Here's the drawing with two shaded views (mm, measured from the low corner). I have some questions. A direction names the side the tool comes from. Coordinates: 2 decimals unless noted, no trailing zeros. Write each loop counter-clockwise with the first axis right and the second up, starting at its lowest first coordinate (ties: lowest second). Pieces come first, ordered by that corner, then holes. Notation, with made-up numbers: (0.25, 20.5) -> (43.25, 20.5) arc R3 ccw to (43.25, 24.5) -> close; hole circle Ø4 at (33.5, 72). An arc over 180 degrees is marked (long way). Put each result on its own line as item: value.
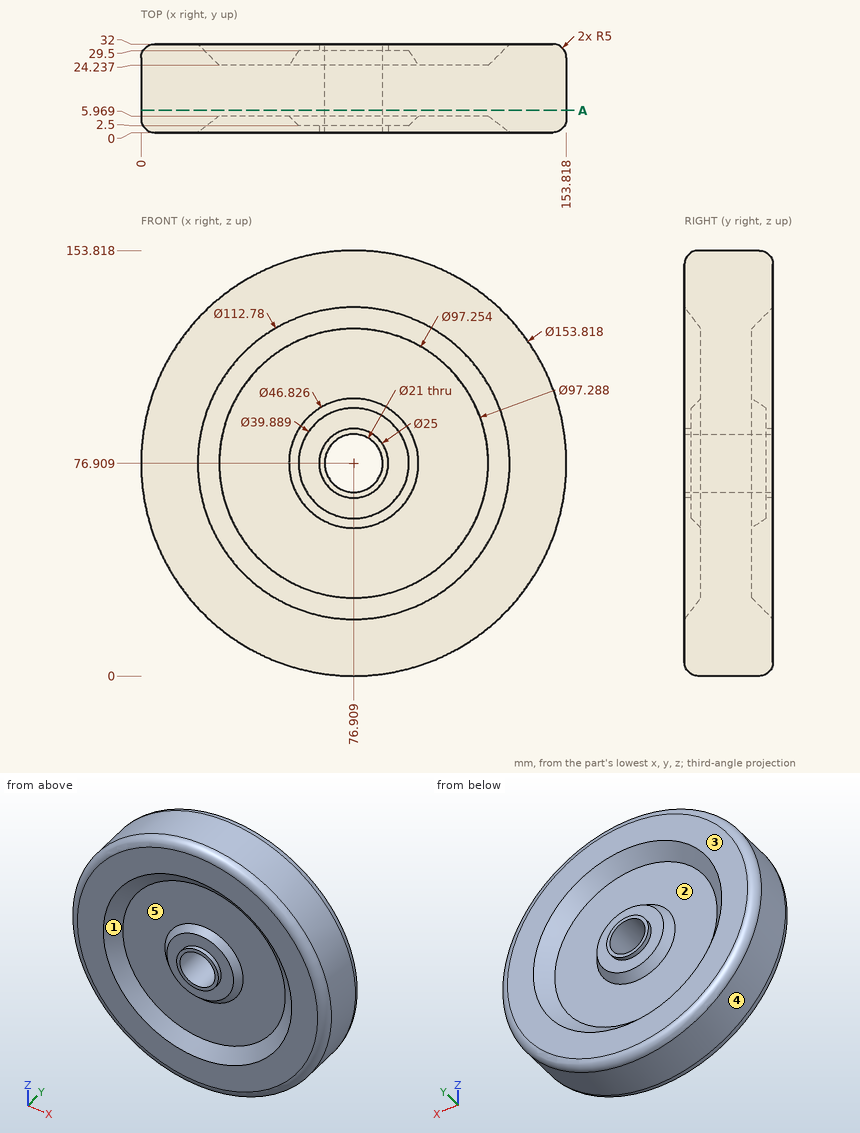
Item 1: Please list where these lines run through material, in increasing order: line 1 along X through (y, z) = (12.5, 76) (1 decimal); line 2 along X through (y, z) = (3.5, 66) (1 decimal); line 3 along Y through (x, z) = (100, 44.5). Write a range as from..to.
Output:
line 1: x = 0..66.4, 87.4..153.8
line 2: x = 1..26.2, 59..94.8, 127.6..152.8
line 3: y = 5.97..24.24
Item 2: Which directions (+Z, -Z, +X, -X, +Y, -Y) give clear straight access to the entire face, cutting with the end or side of a thin tool? Please do the marked faces 1 and 2.
Output:
face 1: -Y
face 2: +Y
Item 3: Imagine slicing it at A-A on y = 8. Write out the boundary of the cut face in (x, z).
Output:
outline: circle Ø153.82 at (76.91, 76.91); hole circle Ø21 at (76.91, 76.91)
Item 4: For P1, Ø8, axis at x = 105.5, y = 6, coming from the +Z side; P2, Ø20, axis at x = 76, z = 72.5, coming from the +Y side; P3, Ø8, axis at y = 21, z = 26.5, coming from the -X side; P4, Ø5, axis at x = 52, y = 22, coming from the +Z side, each with a flat end and sliding along its axis, tell me the tip position at first contact or that it passes through.
Output:
P1: stops at z = 149.78
P2: stops at y = 32
P3: stops at x = 15.58
P4: stops at z = 150.48
Item 5: If we mould it in two halves opening along X, with no side actions, what happens to the marked faces 3, 4 and 5? For each: released by +X, released by -X, zero draft, split by the parting line, or undercut.
Output:
face 3: zero draft
face 4: split by the parting line
face 5: undercut
